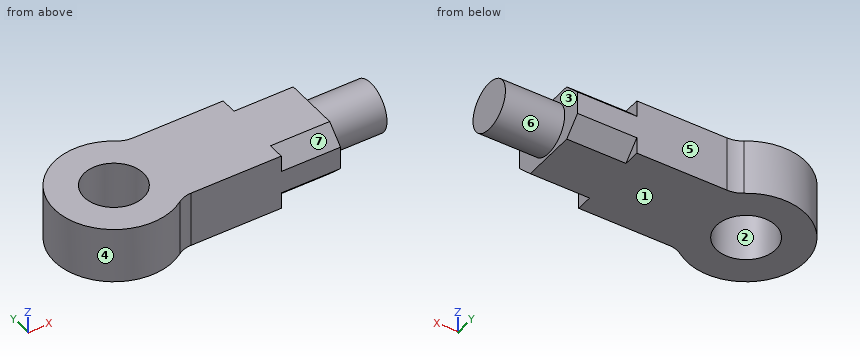
```python
from build123d import *

# Parameters (mm, degrees)
SKETCH1_R           = 6
BOSS_EXTRUDE1_DEPTH = 5.655
BOSS_EXTRUDE2_DEPTH = 12
SKETCH3_R           = 5
BOSS_EXTRUDE3_DEPTH = 12


with BuildPart() as part:
    # Sketch1 → Boss-Extrude1 (new, symmetric)
    with BuildSketch(Plane.XY):
        with BuildLine():
            Line((9.724056813, 8.94427191), (28, 8.94427191))
            Line((28, 8.94427191), (28, -8.94427191))
            Line((28, -8.94427191), (9.724056813, -8.94427191))
            ThreePointArc((9.724056813, -8.94427191), (8.225104215, -9.174246636), (6.864040103, -9.843015466))
            ThreePointArc((6.864040103, -9.843015466), (-12, 0), (6.864040103, 9.843015466))
            ThreePointArc((6.864040103, 9.843015466), (8.225104215, 9.174246636), (9.724056813, 8.94427191))
        make_face()
        Circle(SKETCH1_R, mode=Mode.SUBTRACT)
    extrude(amount=BOSS_EXTRUDE1_DEPTH, both=True)

    # Sketch2 → Boss-Extrude2 (add)
    with BuildSketch(Plane(origin=(28, 0, 0), x_dir=(0, 0, -1), z_dir=(1, 0, 0))):
        Polygon((2.321666667, 8.94427191), (-2.321666667, 8.94427191), (-5.655, 5.610938577), (-5.655, -5.610938577), (-2.321666667, -8.94427191), (2.321666667, -8.94427191), (5.655, -5.610938577), (5.655, 5.610938577), align=None)
    extrude(amount=BOSS_EXTRUDE2_DEPTH)

    # Sketch3 → Boss-Extrude3 (add)
    with BuildSketch(Plane(origin=(40, 0, 0), x_dir=(0, 0, -1), z_dir=(1, 0, 0))):
        Circle(SKETCH3_R)
    extrude(amount=BOSS_EXTRUDE3_DEPTH)


solid = part.part
```
Input: part model. Units: mm. Frame: model coordinates. Face numbers are marked on the shaded views. A direction names the side the tool comes from. Give positions to 0.01 mm unless a question says otherwise; leave off trailing zeros. Loops run counter-clockwise (first coordinate to the right, second up) from the corner with the lowest first, then second, coordinate; pieces in that order, holes last.
1) Mould query, pull axis X, two halves, no side actions, for the marked faces 1, 2, 3 and 4. Classes: released by +X, released by -X, zero draft, split by the parting line, or undercut.
A:
face 1: zero draft
face 2: undercut
face 3: released by +X
face 4: split by the parting line
2) Reachability of the marked faces 5, 6 and 7 from +Z, -Z, +X, -X, +Y, -Y: full face, straight path, thin tool, end or side. Return the list, or none.
A:
face 5: +Z, -Z, +X, +Y
face 6: +X
face 7: +Z, +X, -Y
3) Section query C-C on z = 0. Return the cut outline in (x, y), and give its area (3 significant figures).
A:
outline: (6.86, -9.84) arc R5 cw to (9.72, -8.94) - (40, -8.94) - (40, -5) - (52, -5) - (52, 5) - (40, 5) - (40, 8.94) - (9.72, 8.94) arc R5 cw to (6.86, 9.84) arc R12 ccw (long way) to start; hole circle Ø12 at (0, 0)
area: 983 mm2
4) Line query: L1, parallel to Y at x = 0, z = 1.25; L2, parallel to Y at x = 13, z = -1; L3, parallel to Y at x = -3.5, z = -0.75. Output: solid intervals per line, ascending.
A:
L1: y = -12 to -6, 6 to 12
L2: y = -8.94 to 8.94
L3: y = -11.48 to -4.87, 4.87 to 11.48
5) Section query A-A on x = 0. Return the cut outline in (y, z) (3 decimals).
A:
outline: (-12, -5.655) - (-6, -5.655) - (-6, 5.655) - (-12, 5.655) - close; (6, -5.655) - (12, -5.655) - (12, 5.655) - (6, 5.655) - close
6) Section query D-D on y = -6.75. Return the cut outline in (x, z) (3 decimals), and give its area (3 significant figures).
A:
outline: (-9.922, -5.655) - (28, -5.655) - (28, -4.516) - (40, -4.516) - (40, 4.516) - (28, 4.516) - (28, 5.655) - (-9.922, 5.655) - close
area: 537 mm2
7) Contact query for flat-ended pins moving along their axis: pin 1 (3.5 mm diameter, centred on y = 7, z = 3.5, fed in from +X); pin 2 (3 mm diameter, centred on x = 24, z = 2, fed in from +Y); pin 3 (1.5 mm diameter, centred on x = 17.5, z = -2.5, fed in from -Y). Output: stop coordinate, or through.
A:
pin 1: stops at x = 40
pin 2: stops at y = 8.94
pin 3: stops at y = -8.94
8) Section query B-B on y = 0. Return the cut outline in (x, z) (3 decimals), and give its area (3 significant figures).
A:
outline: (-12, -5.655) - (-6, -5.655) - (-6, 5.655) - (-12, 5.655) - close; (6, -5.655) - (40, -5.655) - (40, -5) - (52, -5) - (52, 5) - (40, 5) - (40, 5.655) - (6, 5.655) - close
area: 572 mm2
